Could you check a few things on this model? Use its own coordinates, in mm. Face numbers are marked on the shaded views. A direction names the side the tool comes from. Give positions to 0.01 mm unless a question says otherwise; leave off trailing zeros. Write each loop counter-clockwise with the first axis right and the second up, starting at its lowest first coordinate (ties: lowest second). Pieces come first, ordered by that corner, then holes. Notation, with made-up numbers: (29, -26) -> (77, -26) arc R18 cw to (77, -15) -> close; hole circle Ø6 at (80.25, 80). An arc over 180 degrees is marked (long way). Write item = value, one per line. Start each with the question number.
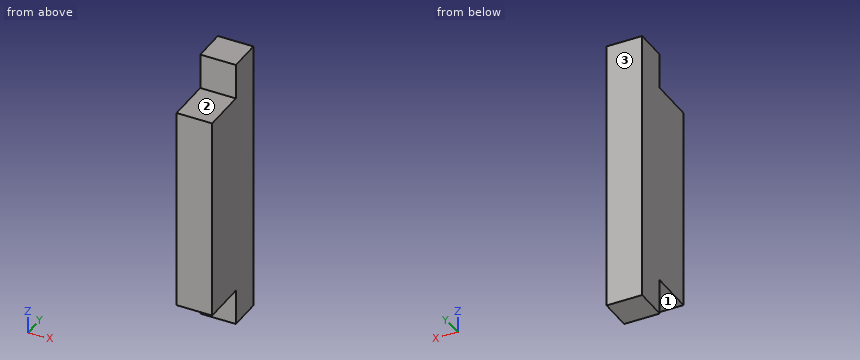
```python
from build123d import *

# Parameters (mm, degrees)
SKETCH1_W           = 29.21
SKETCH1_H           = 11.176
SKETCH1_W_2         = 5.08
SKETCH1_H_2         = 4.7625
BOSS_EXTRUDE1_DEPTH = 5.08


with BuildPart() as part:
    # Sketch1 → Boss-Extrude1 (new body)
    with BuildSketch(Plane(origin=(0, 0, 0), x_dir=(0, 0, -1), z_dir=(1, 0, 0))):
        Rectangle(SKETCH1_W, SKETCH1_H)
        Polygon((-14.605, 0.8255), (-14.605, -5.588), (14.605, -5.588), (14.605, 0.8255), (14.605, 5.588), (-14.605, 5.588), align=None)
        with Locations((-17.145, 3.20675)):
            Rectangle(SKETCH1_W_2, SKETCH1_H_2)
        with Locations((17.145, 3.20675)):
            Rectangle(SKETCH1_W_2, SKETCH1_H_2)
    extrude(amount=BOSS_EXTRUDE1_DEPTH)


solid = part.part
```
(1) Imagine slicing it at B-B (z = 15.5). Please give me the cut outline in (x, y).
(2) If I drill on line 1 along Z through (x, y) = (2.6, -5) (3 decimals); line 2 along Y through (x, z) = (2.9, 16), over which ranges is the centre line in solid material (lowest first)? Write a range as from..to.
(3) Imagine slicing it at C-C (y = 0). Please give me the cut outline in (x, z) (3 decimals), then the cut area to 3 significant figures.
(4) On a 3-axis mill with a long thin cutter (end or side, diameter ignored), from which of +Z, -Z, +X, -X, +Y, -Y can I reach the whole of each face in a straight line? I mean the marked faces 1, 2 and 3. Say none if no direction works.
(5) I'm going to push a flat-ended pin straight in: pin 1 (2.5 mm diameter, centred on x = 3, z = -17.5, fed in from -Y). Where does the tip first touch, or does it pass through?
(6) Imagine slicing it at A-A (x = 1.8). Please give me the cut outline in (y, z) (1 decimal), then the cut area to 3 significant figures.
Answers below:
q1.outline = (0, 0.83) -> (5.08, 0.83) -> (5.08, 5.59) -> (0, 5.59) -> close
q2.line_1 = -14.605..14.605
q2.line_2 = 0.83..5.59
q3.outline = (0, -14.605) -> (5.08, -14.605) -> (5.08, 14.605) -> (0, 14.605) -> close
q3.area = 148 mm^2
q4.face_1 = -Z, +X, -X, -Y
q4.face_2 = +Z, +X, -X, -Y
q4.face_3 = +Z, -Z, +X, -X, +Y
q5.pin_1 = 0.83
q6.outline = (-5.6, -14.6) -> (0.8, -14.6) -> (0.8, -19.7) -> (5.6, -19.7) -> (5.6, 19.7) -> (0.8, 19.7) -> (0.8, 14.6) -> (-5.6, 14.6) -> close
q6.area = 375 mm^2
